Design review of the part shown in the three views and the two pictorial views. Dimensions are in mm from the part's minimum x, y and z. A direction names the side the tool comes from. Coordinates: 2 decimals unless noted, no trailing zeros. Loops run counter-clockwise (first coordinate to the right, second up) from the corner with the lowest first, then second, coordinate; pieces in that order, holes last. Notation, with made-up numbers: (-9.5, -33) -> (30.5, -33) arc R34 cw to (30.5, 6) -> close; hole circle Ø2 at (2, -33.5). An arc over 180 degrees is marked (long way). One line per item, written item: value.
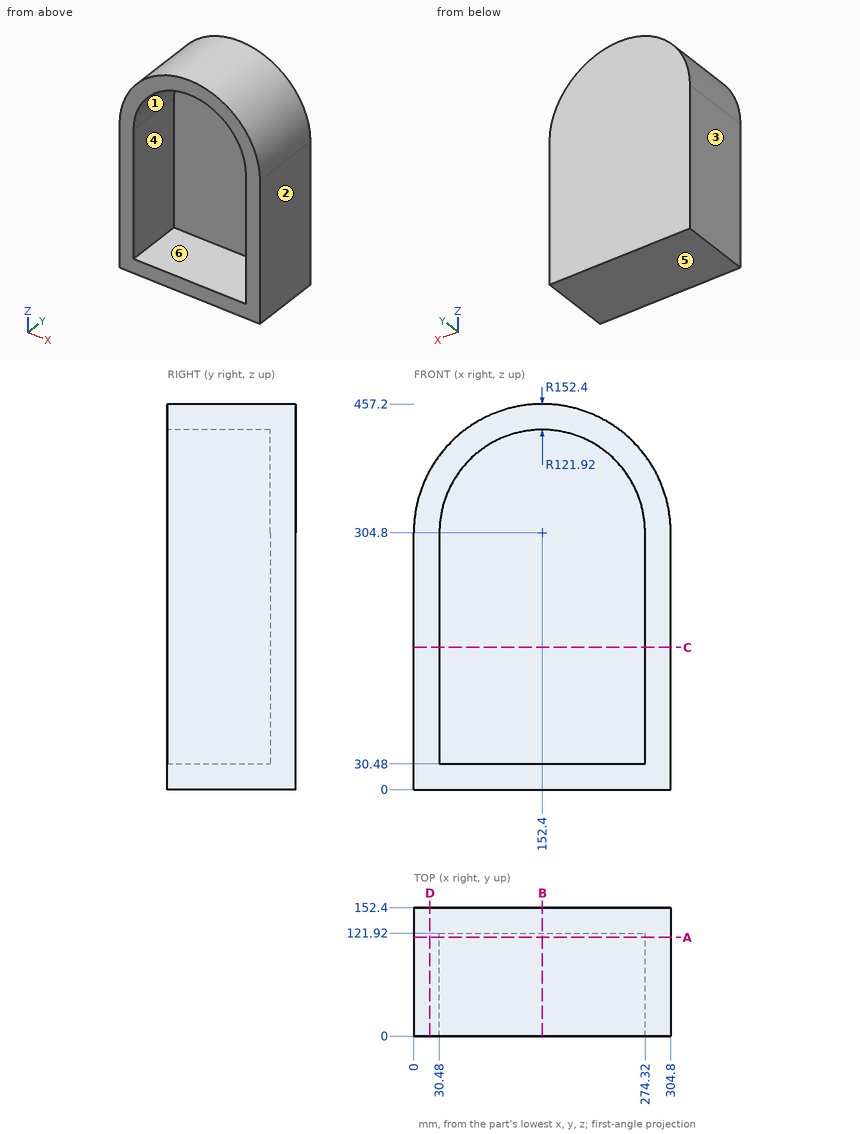
1. To check wall thickness, follow probe 1 along X at (y, z) = (31, 53); probe 2 along Y at (x, z) = (150, 242); probe 3 along Z at (x, y) = (263, 77.5). State the ranges of each line that lie inside material, in increasing order. Write a range as from..to.
Return value:
probe 1: x = 0..30.48, 274.32..304.8
probe 2: y = 121.92..152.4
probe 3: z = 0..30.48, 356.1..409.65
2. Take a section at B-B, the plane x = 152.4. Give the boundary of the cut face in (y, z).
Return value:
outline: (0, 0) -> (152.4, 0) -> (152.4, 457.2) -> (0, 457.2) -> (0, 426.72) -> (121.92, 426.72) -> (121.92, 30.48) -> (0, 30.48) -> close
3. Take a section at D-D, the plane x = 19. Give the boundary of the cut face in (y, z), and give its area (3 significant figures).
Return value:
outline: (0, 0) -> (152.4, 0) -> (152.4, 378.49) -> (0, 378.49) -> close
area: 57,700 mm2
4. Insertion check: pin 1 Ø1.5 at (x, z) = (104.5, 196) entering from -Y. The pin has a flat end and moves straight along its axis. Give the tip position at first contact, or say it passes through.
Return value:
pin 1: stops at y = 121.92
5. The part is to be moulded in two halves that separate along Z. For the marked faces 3, 4, 5 and 6, say which applies: pulls with the +Z half, pulls with the -Z half, needs draft (parallel to the pull), parting line crosses it, or undercut.
Return value:
face 3: needs draft
face 4: undercut
face 5: pulls with the -Z half
face 6: undercut
6. Take a section at A-A, the plane y = 117. Give the boundary of the cut face in (x, z), and give its area (3 significant figures).
Return value:
outline: (0, 0) -> (304.8, 0) -> (304.8, 304.8) arc R152.4 ccw to (0, 304.8) -> close; hole (30.48, 30.48) -> (274.32, 30.48) -> (274.32, 304.8) arc R121.92 ccw to (30.48, 304.8) -> close
area: 39,100 mm2
7. For the marked faces 1 and 2, list the 3-axis set-ups (+Z, -Z, +X, -X, +Y, -Y) from which the entire face can be reached by the end or side of a thin tool; tool diameter is ignored.
Return value:
face 1: -Y
face 2: +Z, -Z, +X, +Y, -Y
8. Take a section at C-C, the plane z = 168.5. Give the boundary of the cut face in (x, y), and give its area (3 significant figures).
Return value:
outline: (0, 0) -> (30.48, 0) -> (30.48, 121.92) -> (274.32, 121.92) -> (274.32, 0) -> (304.8, 0) -> (304.8, 152.4) -> (0, 152.4) -> close
area: 16,700 mm2
